Read the model definition and answer for the solid it produces. Units are mm, in the model's axes. Face numbers are marked on the shaded views. A direction names the side the tool comes from. Give positions to 0.01 mm unless a question says otherwise; leave off trailing zeros. Order: outer loops, then holes, each group sorted by start corner. A loop starts at its lowest first (then second) coordinate and runs counter-clockwise, first axis right, second up. Notation, with made-up numbers: (14, 22) - (58, 22) arc R37 ccw to (58, 61) - close; hole circle Ø3 at (56.25, 14.25). An arc over 180 degrees is marked (long way). Write item = value, one per line.
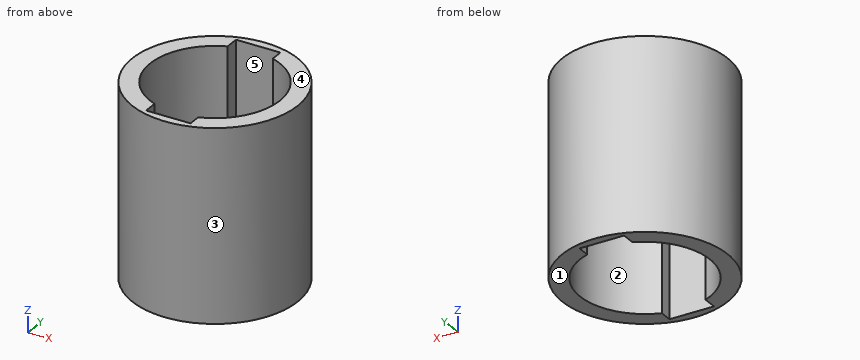
```python
from build123d import *

# Parameters (mm, degrees)
SKETCH1_R           = 6.5
BOSS_EXTRUDE1_DEPTH = 15
CUT_EXTRUDE1_DEPTH  = 18.592612086


with BuildPart() as part:
    # Sketch1 → Boss-Extrude1 (new body)
    with BuildSketch(Plane(origin=(0, 0, 0), x_dir=(0, 1, 0), z_dir=(0, 0, 1))):
        with Locations(Location((0, 0, 0), (0, 0, 270))):
            Circle(SKETCH1_R)
    extrude(amount=BOSS_EXTRUDE1_DEPTH)

    # Sketch2 → Cut-Extrude1 (cut, through all)
    with BuildSketch(Plane.XY.offset(15)):
        with BuildLine():
            Line((-1.886299685, 4.738340796), (-1.886299685, 5.838340796))
            Line((-1.886299685, 5.838340796), (1.612593669, 5.838340796))
            Line((1.612593669, 5.838340796), (1.612593669, 4.838340796))
            ThreePointArc((1.612593669, 4.838340796), (5.1, 0), (1.612593669, -4.838340796))
            Line((1.612593669, -4.838340796), (1.612593669, -5.838340796))
            Line((1.612593669, -5.838340796), (-1.886299685, -5.838340796))
            Line((-1.886299685, -5.838340796), (-1.886299685, -4.738340796))
            ThreePointArc((-1.886299685, -4.738340796), (-5.1, 0), (-1.886299685, 4.738340796))
        make_face()
    extrude(amount=-CUT_EXTRUDE1_DEPTH, mode=Mode.SUBTRACT)


solid = part.part
```
1. Section C-C (z = 5.75) is taken. Determine the outline of the cut face in (x, y), and give its area (3 significant figures).
Recorded:
outline = circle Ø13 at (0, 0); hole (-1.89, -5.84) - (1.61, -5.84) - (1.61, -4.84) arc R5.1 ccw to (1.61, 4.84) - (1.61, 5.84) - (-1.89, 5.84) - (-1.89, 4.74) arc R5.1 ccw to (-1.89, -4.74) - close
area = 45.1 mm^2
2. Straight lines are drawn through the part: L1, parallel to Y at x = 4.5, z = 11.25; L2, parallel to X at y = 5.75, z = 7; L3, parallel to Y at x = 0.25, z = 3.25. For each, find the intervals that lie inside material, in ascending order. Write a range as [from, to].
Recorded:
L1 = [-4.69, -2.4], [2.4, 4.69]
L2 = [-3.03, -1.89], [1.61, 3.03]
L3 = [-6.5, -5.84], [5.84, 6.5]
3. For the marked faces 4 and 5, determine the directions among +Z, -Z, +X, -X, +Y, -Y from which every point of the face is accessible in a straight line to the end or side of a thin tool.
Recorded:
face_4 = +Z, +X, -X, +Y, -Y
face_5 = +Z, -Z
4. Section A-A (x = 0) is taken. Determine the outline of the cut face in (y, z), and give its area (3 significant figures).
Recorded:
outline = (-6.5, 0) - (-5.84, 0) - (-5.84, 15) - (-6.5, 15) - close; (5.84, 0) - (6.5, 0) - (6.5, 15) - (5.84, 15) - close
area = 19.8 mm^2
5. Section B-B (y = 0) is taken. Determine the outline of the cut face in (x, z), and give its area (3 significant figures).
Recorded:
outline = (-6.5, 0) - (-5.1, 0) - (-5.1, 15) - (-6.5, 15) - close; (5.1, 0) - (6.5, 0) - (6.5, 15) - (5.1, 15) - close
area = 42.0 mm^2
6. Flat-ended cylindrical pins translate along their axes: pin 1 (2 mm diameter, centred on x = 2.5, z = 12.5, fed in from +Y); pin 2 (6 mm diameter, centred on x = 4, z = 6, fed in from -Y); pin 3 (1 mm diameter, centred on y = -1, z = 10, fed in from -X); pin 4 (1 mm diameter, centred on x = 2, y = 2, fed in from -Z). Find the tip coordinate at first contact, or state that the pin passes through.
Recorded:
pin_1 = 6.32
pin_2 = -6.42
pin_3 = -6.48
pin_4 = through
7. Determine the mould class of the marked faces 1, 2 and 3 for opening direction X: +X half, -X half, draft (parallel to the pull), parting line (faces both ways), or undercut.
Recorded:
face_1 = draft
face_2 = undercut
face_3 = parting line
